Source: CAD feature listing. Evaluate the final solid. Frame: model axes, mm. Round coordinates to 2 decimals unless told otherwise and drop trailing zeros. Loops run counter-clockwise (first coordinate to the right, second up) from the corner with the lowest first, then second, coordinate; pieces in that order, holes last.
Item 1: Section query A-A on x = 208. Return loops of the section in (y, z), then the cut area to 3 significant figures.
Item 2: Section query C-C on z = -25. Return loops of the section in (x, y), then the cut area to 3 significant figures.
Item 3: Ray query, L1, parallel to X at y = -951, z = -24; L2, parallel to Y at x = -122, z = -5.5. Return the intervals inside material, ascending.
Item 4: First-contact query: P1, Ø8, axis at x = 219.5, z = -20.5, coming from the -Y side. Flat tip, straight axial feed; report the tip coordinate or a pass-through.
Item 5: Section query B-B on y = 118.5. Return loops of the section in (x, z), then the cut area to 3 significant figures.
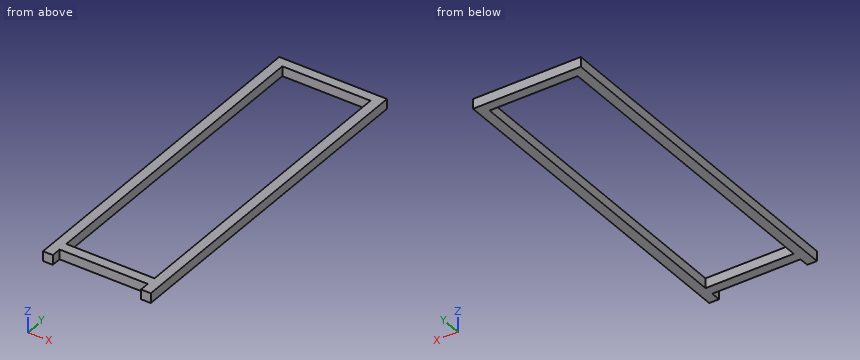
```python
from build123d import *

# Parameters (mm, degrees)
CROQUIS1_W              = 450
CROQUIS1_H              = 1600
SALIENTE_EXTRUIR1_DEPTH = 50


with BuildPart() as part:
    # Croquis1 → Saliente-Extruir1 (new body)
    with BuildSketch(Plane.XY):
        Polygon((-275, -1500), (-275, 250), (275, 250), (275, -1500), (225, -1500), (225, -1450), (-225, -1450), (-225, -1500), align=None)
        with Locations((0, -600)):
            Rectangle(CROQUIS1_W, CROQUIS1_H, mode=Mode.SUBTRACT)
    extrude(amount=-SALIENTE_EXTRUIR1_DEPTH)


solid = part.part
```
Data:
1. outline: (-1450, -50) - (-1400, -50) - (-1400, 0) - (-1450, 0) - close; (200, -50) - (250, -50) - (250, 0) - (200, 0) - close
1. area: 5,000 mm2
2. outline: (-275, -1500) - (-225, -1500) - (-225, -1450) - (225, -1450) - (225, -1500) - (275, -1500) - (275, 250) - (-275, 250) - close; hole (-225, -1400) - (225, -1400) - (225, 200) - (-225, 200) - close
2. area: 220,000 mm2
3. L1: x = -275 to -225, 225 to 275
3. L2: y = -1450 to -1400, 200 to 250
4. P1: stops at y = -1450
5. outline: (-275, -50) - (-225, -50) - (-225, 0) - (-275, 0) - close; (225, -50) - (275, -50) - (275, 0) - (225, 0) - close
5. area: 5,000 mm2
